```python
from build123d import *

# Parameters (mm, degrees)
F0_W     = 102
F0_H     = 102
F1_DEPTH = 4
F2_W     = 102
F2_H     = 102
F2_W_2   = 100
F2_H_2   = 100
F3_DEPTH = 35
F4_W     = 81.75
F4_H     = 81.75
F4_W_2   = 79.75
F4_H_2   = 79.75
F5_DEPTH = 15
F7_DEPTH = 10


# Not quite as in the source:
# - a feature names something its author has since deleted; it is built from what else it names


with BuildPart() as f1:
    # F0 (on Top) → F1 (new body)
    with BuildSketch(Plane.XY):
        Rectangle(F0_W, F0_H)
    extrude(amount=F1_DEPTH)

    # F2 (on Top) → F3 (join)
    with BuildSketch(Plane.XY):
        Rectangle(F2_W, F2_H)
        Rectangle(F2_W_2, F2_H_2, mode=Mode.SUBTRACT)
    extrude(amount=F3_DEPTH)

    # F4 (on Top) → F5 (join)
    with BuildSketch(Plane.XY):
        Rectangle(F4_W, F4_H)
        Rectangle(F4_W_2, F4_H_2, mode=Mode.SUBTRACT)
    extrude(amount=F5_DEPTH)

    # F6: union 

    # F7 (add): a face of the model
    f7_faces = [f1.faces().sort_by_distance(p)[0] for p in [
        (0, 0, 4),
    ]]
    extrude(f7_faces, amount=F7_DEPTH)


solid = f1.part
```
Can you work these out from the model? Positions are in its coordinate system, mm. A direction names the side the tool comes from. Coordinates: 2 decimals unless noted, no trailing zeros. Write each loop counter-clockwise with the first axis right and the second up, starting at its lowest first coordinate (ties: lowest second). Pieces come first, ordered by that corner, then holes. Notation, with made-up numbers: (45.5, 46) - (72.5, 46) arc R7 ccw to (72.5, 53) - close; hole circle Ø7 at (40.25, 20.5). An arc over 180 degrees is marked (long way). Return JSON: item names as keys, results as strings.
Q1. If we section it at A-A (z = 12): Please give me the cut outline in (x, y) (3 decimals).
Computed values:
{"outline": "(-51, -51) - (51, -51) - (51, 51) - (-51, 51) - close; (-40.875, -40.875) - (40.875, -40.875) - (40.875, 40.875) - (-40.875, 40.875) - close; hole (-50, -50) - (50, -50) - (50, 50) - (-50, 50) - close"}
Q2. Thinking about a two-plate mould opening in Y: for faces 1 (the flat face through (-1, 40.875, 9)), 2 (the flat face through (-1, 51, 17)), 3 (the flat face through (51, -1, 17)), 4 (the flat face through (-45, 1, 4)), which applies, +Y half, -Y half, draft (parallel to the pull), parting line (faces both ways), or undercut?
Computed values:
{"face 1": "undercut", "face 2": "+Y half", "face 3": "draft", "face 4": "undercut"}
Q3. Please list where these lines run through material, in increasing order: L1, parallel to X at y = 3, z = 9 (3 decimals); L2, parallel to Y at x = -5.5, z = 17. Write a range as from..to.
Computed values:
{"L1": "x = -51..-50, -40.875..40.875, 50..51", "L2": "y = -51..-50, 50..51"}
Q4. On a 3-axis mill with a long thin cutter (end or side, diameter ignored), from which of +Z, -Z, +X, -X, +Y, -Y can I reach the whole of each face in a straight line? I mean faces 5 (the flat face through (-1, -50, 19)), 6 (the flat face through (-1, -51, 17)). Say none if no direction works.
Computed values:
{"face 5": "+Z", "face 6": "+Z, -Z, +X, -X, -Y"}
Q5. If we section it at C-C (z = 21): Please give me the cut outline in (x, y).
Computed values:
{"outline": "(-51, -51) - (51, -51) - (51, 51) - (-51, 51) - close; hole (-50, -50) - (50, -50) - (50, 50) - (-50, 50) - close"}
Q6. I'm going to push flat-ended pins straight in: pin 1 Ø4 at (x, y) = (0.5, 4) entering from +Z; pin 2 Ø8 at (x, y) = (-1, 38.5) entering from +Z. Where does each tip first touch, or does it pass through?
Computed values:
{"pin 1": "stops at z = 14", "pin 2": "stops at z = 15"}
Q7. If we section it at B-B (x = -24): Please give me the cut outline in (y, z) (3 decimals), then the cut area to 3 significant figures.
Computed values:
{"outline": "(-51, 0) - (51, 0) - (51, 35) - (50, 35) - (50, 4) - (40.875, 4) - (40.875, 15) - (39.875, 15) - (39.875, 14) - (-39.875, 14) - (-39.875, 15) - (-40.875, 15) - (-40.875, 4) - (-50, 4) - (-50, 35) - (-51, 35) - close", "area": "1,290 mm2"}
